```python
from build123d import *

# Parameters (mm, degrees)
F0_W     = 73
F0_H     = 59
F1_DEPTH = 5
F2_SIZE  = 25
F4_D     = 3.3
F4_DEPTH = 13.8
F4_TIP   = 0.9914200214
F3_R     = 13.4455987062
F5_DEPTH = 5


with BuildPart() as f1:
    # F0 (on Top) → F1 (new body)
    with BuildSketch(Plane.XY):
        Rectangle(F0_W, F0_H)
        with BuildLine():
            Line((-32.5, 13.5), (-32.5, 23.5))
            ThreePointArc((-32.5, 23.5), (-30, 26), (-27.5, 23.5))
            Line((-27.5, 23.5), (-27.5, 13.5))
            ThreePointArc((-27.5, 13.5), (-30, 11), (-32.5, 13.5))
        make_face(mode=Mode.SUBTRACT)
        with BuildLine():
            Line((27.5, 13.5), (27.5, 23.5))
            ThreePointArc((27.5, 23.5), (30, 26), (32.5, 23.5))
            Line((32.5, 23.5), (32.5, 13.5))
            ThreePointArc((32.5, 13.5), (30, 11), (27.5, 13.5))
        make_face(mode=Mode.SUBTRACT)
    extrude(amount=F1_DEPTH)

    # F2
    f2_edges = [f1.edges().sort_by_distance(p)[0] for p in [
        (-36.5, -29.5, 2.5),
        (36.5, -29.5, 2.5),
    ]]
    chamfer(f2_edges, length=F2_SIZE)

    # F4
    with Locations(Plane.XY.offset(5)):
        with Locations((-21.9203102168, -2.5796897832), (0, -24.5), (21.9203102168, -2.5796897832)):
            Hole(F4_D / 2, depth=F4_DEPTH)
            with Locations((0, 0, -(F4_DEPTH + F4_TIP / 2))):  # 118° drill point
                Cone(0, F4_D / 2, F4_TIP, mode=Mode.SUBTRACT)

    # F3 (on face) → F5 (cut, through all)
    with BuildSketch(Plane.XY.offset(5)):
        with Locations((0, -2.5796897832)):
            Circle(F3_R)
    extrude(amount=-F5_DEPTH, mode=Mode.SUBTRACT)


solid = f1.part
```
Verification items for the finished model (mm, model axes). A direction names the side the tool comes from. Give positions to 0.01 mm unless a question says otherwise; leave off trailing zeros. Loops run counter-clockwise (first coordinate to the right, second up) from the corner with the lowest first, then second, coordinate; pieces in that order, holes last.
1. Go/stop test with a flat-tipped pin: pin 1 Ø21.5 at (x, y) = (0, -2.58) entering from +Z. Record where the tip stops, or that it passes through.
2. Thickness scan on line 1 (Y direction, x = 0, z = 3.8); line 2 (X direction, y = -1.5, z = 1.2); line 3 (X direction, y = 24.5, z = 4.55). Record the ranges inside material, lowest first.
3. Set-up check for faces 1 (the cylindrical face through (30, 11, 2)), 2 (the flat face through (-1, 14, 5)): record each of +Z, -Z, +X, -X, +Y, -Y from which the full face is reachable in a straight line by a thin tool's end or side.
4. Section check A-A, the plane x = -30. Enter the section's corners in (y, z), then the cut area to 4 significant figures.
5. Section check D-D, the plane z = 1.65. Enter the section's corners in (x, y).
6. Section check C-C, the plane x = 0. Enter the section's corners in (y, z).
7. Mould release check, pull along Y, two halves, no side actions. Record for faces 3 (the flat face through (-1, 14, 0)), 4 (the flat face through (-27.5, 19, 2)), 5 (the flat face through (-24, -17, 2)): released by +Y, released by -Y, zero draft, split by the parting line, or undercut.
8. Section check B-B, the plane y = -24.5. Enter the section's corners in (x, z), then the cut area to 4 significant figures.
Geometry says:
1. pin 1: passes through
2. line 1: y = -29.5 to -26.15, -22.85 to -16.03, 10.87 to 29.5
2. line 2: x = -36.5 to -23.17, -20.67 to -13.4, 13.4 to 20.67, 23.17 to 36.5
2. line 3: x = -36.5 to -32.29, -27.71 to 27.71, 32.29 to 36.5
3. face 1: +Z, -Z
3. face 2: +Z, +X, -X, +Y, -Y
4. outline: (-11, 0) - (11, 0) - (11, 5) - (-11, 5) - close; (26, 0) - (29.5, 0) - (29.5, 5) - (26, 5) - close
4. area: 127.5 mm2
5. outline: (-36.5, -4.5) - (-11.5, -29.5) - (11.5, -29.5) - (36.5, -4.5) - (36.5, 29.5) - (-36.5, 29.5) - close; hole (-32.5, 13.5) arc R2.5 ccw to (-27.5, 13.5) - (-27.5, 23.5) arc R2.5 ccw to (-32.5, 23.5) - close; hole circle Ø3.3 at (-21.92, -2.58); hole circle Ø26.89 at (0, -2.58); hole circle Ø3.3 at (0, -24.5); hole circle Ø3.3 at (21.92, -2.58); hole (27.5, 13.5) arc R2.5 ccw to (32.5, 13.5) - (32.5, 23.5) arc R2.5 ccw to (27.5, 23.5) - close
6. outline: (-29.5, 0) - (-26.15, 0) - (-26.15, 5) - (-29.5, 5) - close; (-22.85, 0) - (-16.03, 0) - (-16.03, 5) - (-22.85, 5) - close; (10.87, 0) - (29.5, 0) - (29.5, 5) - (10.87, 5) - close
7. face 3: zero draft
7. face 4: undercut
7. face 5: released by -Y
8. outline: (-16.5, 0) - (-1.65, 0) - (-1.65, 5) - (-16.5, 5) - close; (1.65, 0) - (16.5, 0) - (16.5, 5) - (1.65, 5) - close
8. area: 148.5 mm2
